Build history of the part. All positions in model axes, mm. A direction names the side the tool comes from. Round coordinates to 2 decimals unless told otherwise and drop trailing zeros. Write each loop counter-clockwise with the first axis right and the second up, starting at its lowest first coordinate (ties: lowest second). Pieces come first, ordered by that corner, then holes. Notation, with made-up numbers: M 40.25,-28 L 76.25,-28 A22 ccw 76.25,6 Z; hole C 85,-5 d4. An arc over 180 degrees is marked long. Use a Markdown table: item, result.
from build123d import *

# Parameters (mm, degrees)
SKETCH_W        = 36.7
SKETCH_H        = 51.4
SKETCH_W_2      = 31.7
SKETCH_H_2      = 28.6
PAD_DEPTH       = 3
PAD001_DEPTH    = 36.7
SKETCH002_R     = 1.6
POCKET_DEPTH    = 4.501
SKETCH003_W     = 9.5
SKETCH003_H     = 9.5
POCKET001_DEPTH = 1.5
SKETCH004_W     = 36.7
SKETCH004_H     = 31.1
PAD002_DEPTH    = 20
PAD002_FACE31_W = 28.6
PAD002_FACE31_H = 31.7
POCKET002_DEPTH = 20.001
POCKET003_DEPTH = 36.701
FILLET_R        = 3


with BuildPart() as part:
    # Sketch → Pad (new body)
    with BuildSketch(Plane.XY):
        with Locations((0, 15.7)):
            Rectangle(SKETCH_W, SKETCH_H)
        with Locations((0, 24.6)):
            Rectangle(SKETCH_W_2, SKETCH_H_2, mode=Mode.SUBTRACT)
    extrude(amount=PAD_DEPTH)

    # Sketch001 (on Face4 of Pad) → Pad001 (join)
    with BuildSketch(Plane(origin=(-18.35, 0, 0), x_dir=(0, -1, 0), z_dir=(-1, 0, 0))):
        Polygon((-4.75, 0), (4.75, 0), (2.95, -1.5), (-2.95, -1.5), align=None)
    extrude(amount=-PAD001_DEPTH)

    # Sketch002 (on Face16 of Pad001) → Pocket (cut, through all)
    with BuildSketch(Plane(origin=(0, 0, -1.5), x_dir=(1, 0, 0), z_dir=(0, 0, -1))):
        with Locations((-9.175, 0)):
            Circle(SKETCH002_R)
        with Locations((9.175, 0)):
            Circle(SKETCH002_R)
    extrude(amount=-POCKET_DEPTH, mode=Mode.SUBTRACT)

    # Sketch003 (on Face18 of Pocket) → Pocket001 (cut)
    with BuildSketch(Plane(origin=(0, 0, -1.5), x_dir=(1, 0, 0), z_dir=(0, 0, -1))):
        with Locations((-9.175, 0)):
            Rectangle(SKETCH003_W, SKETCH003_H)
        with Locations((9.175, 0)):
            Rectangle(SKETCH003_W, SKETCH003_H)
    extrude(amount=-POCKET001_DEPTH, mode=Mode.SUBTRACT)

    # Sketch004 (on Face4 of Pocket001) → Pad002 (join)
    with BuildSketch(Plane(origin=(0, 0, 0), x_dir=(1, 0, 0), z_dir=(0, 0, -1))):
        with Locations((0, -25.85)):
            Rectangle(SKETCH004_W, SKETCH004_H)
    extrude(amount=PAD002_DEPTH)

    # Pad002 Face31 → Pocket002 (cut, through all)
    with BuildSketch(Plane(origin=(0, 24.6, 0), x_dir=(0, 1, 0), z_dir=(0, 0, 1))):
        Rectangle(PAD002_FACE31_W, PAD002_FACE31_H)
    extrude(amount=-POCKET002_DEPTH, mode=Mode.SUBTRACT)

    # Sketch005 (on Face11 of Pocket002) → Pocket003 (cut, through all)
    with BuildSketch(Plane.YZ.offset(18.35)):
        Polygon((10.3, 0), (10.3, -20), (38.9, -20), align=None)
    extrude(amount=-POCKET003_DEPTH, mode=Mode.SUBTRACT)

    # Fillet
    fillet_edges = [part.edges().sort_by_distance(p)[0] for p in [
        (18.35, 41.4, -10),
        (-18.35, 41.4, -10),
        (-18.35, -10, 1.5),
        (18.35, -10, 1.5),
    ]]
    fillet(fillet_edges, radius=FILLET_R)


solid = part.part
Q1. Cut at D-D on z = -13. Give the cut face in (x, y).
Response values:
| item | result |
|---|---|
| outline | M -18.35,28.89 L -15.85,28.89 L -15.85,38.9 L 15.85,38.9 L 15.85,28.89 L 18.35,28.89 L 18.35,38.4 A3 ccw 15.35,41.4 L -15.35,41.4 A3 ccw -18.35,38.4 Z |
Q2. Cut at C-C on y = 35.5. Give the cut face in (x, z), and give its area (3 significant figures).
Response values:
| item | result |
|---|---|
| outline | M -18.35,-17.62 L -15.85,-17.62 L -15.85,3 L -18.35,3 Z; M 15.85,-17.62 L 18.35,-17.62 L 18.35,3 L 15.85,3 Z |
| area | 103 mm2 |
Q3. Two-plate mould, pull along X, no slides. Class faces 4 (the flat face through (-0.06, 3.84, -0.76)), 5 (the cylindrical face through (-7.65, -0.48, 1.48)), 6 (the cylindrical face through (17.45, 40.54, -8.66)): +X half, -X half, draft (parallel to the pull), parting line (faces both ways), or undercut.
Response values:
| item | result |
|---|---|
| face 4 | draft |
| face 5 | undercut |
| face 6 | +X half |
Q4. Drop flat-ended pins along their axis: P1, Ø6, axis at x = -6, y = 4, coming from the -Z side; P2, Ø12, axis at x = 11.5, y = 29, coming from the +Z side; P3, Ø11.5, axis at x = 3.5, z = -7.5, coming from the -Y side; P4, Ø6, axis at x = 8.5, y = -4, coming from the -Z side. Give the stop position or say it passes through.
Response values:
| item | result |
|---|---|
| P1 | stops at z = -1.5 |
| P2 | stops at z = 3 |
| P3 | stops at y = 38.9 |
| P4 | stops at z = 0 |
Q5. Which spindle directions (+Z, -Z, +X, -X, +Y, -Y) get a long thin tool onto all of the face, cutting with end or side? Do faces 1 (the flat face through (-16.17, 3.84, -0.76)), 2 (the flat face through (16, 0, -1.5)), 3 (the flat face through (0, 10.3, 1)). Say none if no direction does.
Response values:
| item | result |
|---|---|
| face 1 | -Z, +X, -X |
| face 2 | -Z, +X, -X, -Y |
| face 3 | +Z, -Z |
Q6. Cut at B-B on y = 0. Give the cut face in (x, z) (3 decimals).
Response values:
| item | result |
|---|---|
| outline | M -18.35,-1.5 L -13.925,-1.5 L -13.925,0 L -10.775,0 L -10.775,3 L -18.35,3 Z; M -7.575,0 L -4.425,0 L -4.425,-1.5 L 4.425,-1.5 L 4.425,0 L 7.575,0 L 7.575,3 L -7.575,3 Z; M 10.775,0 L 13.925,0 L 13.925,-1.5 L 18.35,-1.5 L 18.35,3 L 10.775,3 Z |
Q7. Cut at A-A on x = -12. Give the cut face in (y, z).
Response values:
| item | result |
|---|---|
| outline | M -10,0 L 10.3,0 L 10.3,3 L -10,3 Z; M 38.9,-20 L 41.4,-20 L 41.4,3 L 38.9,3 Z |
Q8. Drill centre lines: L1, parallel to X at y = 0, z = 2.35 (3 decimals); L2, parallel to X at y = 35, z = -10.5; L3, parallel to Y at x = -3.5, z = 0.25. Where is each one in solid material? Low to high.
Response values:
| item | result |
|---|---|
| L1 | x = -18.35 to -10.775, -7.575 to 7.575, 10.775 to 18.35 |
| L2 | x = -18.35 to -15.85, 15.85 to 18.35 |
| L3 | y = -10 to 10.3, 38.9 to 41.4 |
